Check sheet for the modelled part. Datum: model origin and axes. Units: mm. Face numbers are marked on the shaded views. A direction names the side the tool comes from. Round coordinates to 2 decimals unless told otherwise and drop trailing zeros. Write each loop counter-clockwise with the first axis right and the second up, starting at its lowest first coordinate (ties: lowest second). Pieces come first, ordered by that corner, then holes. Notation, with made-up numbers: M -12.75,64 L 7.25,64 A15 ccw 7.25,84 Z; hole C 52.25,-15 d1. An arc over 180 degrees is marked long. One line per item, written item: value.
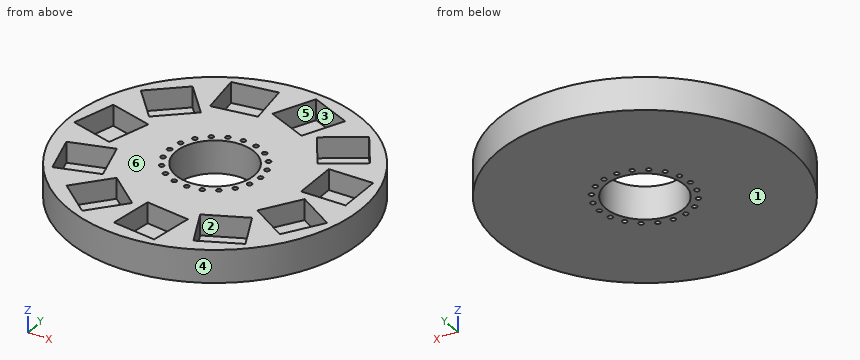
Autodesk Inventor part; units mm, degrees
ref_plane "YZ Plane" through (0, 0, 0) normal (1, 0, 0) x (0, 1, 0)
ref_plane "XZ Plane" through (0, 0, 0) normal (0, 1, 0) x (-1, 0, 0)
ref_plane "XY Plane" through (0, 0, 0) normal (0, 0, 1) x (1, 0, 0)
sketch "Sketch1" plane through (0, 0, 0) normal (0, 0, 1) x (1, 0, 0)
  circle A0 centre (0, 0) radius 45
  circle A1 centre (0, 0) radius 12
  dimension "d0" = 90
  dimension "d1" = 24
extrude "Extrusion1" add sketch "Sketch1" along normal blind 10
sketch "Sketch2" plane through (0, 0, 10) normal (0, 0, 1) x (1, 0, 0)
  line L0 (27.3, 12.7) -> (40, 12.7)
  line L1 (40, 12.7) -> (40, 0)
  line L2 (40, 0) -> (27.3, 0)
  line L3 (27.3, 0) -> (27.3, 12.7)
  line L4 (40.5, 13.2) -> (26.8, 13.2)
  line L5 (26.8, 13.2) -> (26.8, -0.5)
  line L6 (26.8, -0.5) -> (40.5, -0.5)
  line L7 (40.5, -0.5) -> (40.5, 13.2)
  point P0 (0, 0)
  dimension "d4" = 12.7
  dimension "d5" = 12.7
  dimension "d6" = 40
  dimension "d7" = 0.5
extrude "Extrusion2" cut sketch "Sketch2" against normal blind 6.35 contours L0 L1 L2 L3 | L7 L6 L5 L4
pattern_circular "Circular Pattern1" count 11 over 360 about axis through (0, 0, 0) along (0, 0, 1) of "Extrusion2"
sketch "Sketch3" plane through (0, 0, 10) normal (0, 0, 1) x (1, 0, 0)
  circle A0 centre (20, 0) radius 1.75
  circle A1 centre (14.1421, 14.1421) radius 1.75
  circle A2 centre (0, 20) radius 1.75
  circle A3 centre (-14.1421, 14.1421) radius 1.75
  circle A4 centre (-20, 0) radius 1.75
  circle A5 centre (-14.1421, -14.1421) radius 1.75
  circle A6 centre (0, -20) radius 1.75
  circle A7 centre (14.1421, -14.1421) radius 1.75
  point P0 (0, 0)
  dimension "d13" = 3.5
  dimension "d14" = 20
  dimension "d17" = 360
extrude "Extrusion3" [suppressed]
sketch "Sketch6" plane through (0, 0, 0) normal (0, 0, -1) x (-1, 0, 0)
  circle A0 centre (0, 14) radius 0.75
  circle A1 centre (-4.3262, 13.3148) radius 0.75
  circle A2 centre (-8.229, 11.3262) radius 0.75
  circle A3 centre (-11.3262, 8.229) radius 0.75
  circle A4 centre (-13.3148, 4.3262) radius 0.75
  circle A5 centre (-14, 0) radius 0.75
  circle A6 centre (-13.3148, -4.3262) radius 0.75
  circle A7 centre (-11.3262, -8.229) radius 0.75
  circle A8 centre (-8.229, -11.3262) radius 0.75
  circle A9 centre (-4.3262, -13.3148) radius 0.75
  circle A10 centre (0, -14) radius 0.75
  circle A11 centre (4.3262, -13.3148) radius 0.75
  circle A12 centre (8.229, -11.3262) radius 0.75
  circle A13 centre (11.3262, -8.229) radius 0.75
  circle A14 centre (13.3148, -4.3262) radius 0.75
  circle A15 centre (14, 0) radius 0.75
  circle A16 centre (13.3148, 4.3262) radius 0.75
  circle A17 centre (11.3262, 8.229) radius 0.75
  circle A18 centre (8.229, 11.3262) radius 0.75
  circle A19 centre (4.3262, 13.3148) radius 0.75
  point P0 (0, 0)
  dimension "d24" = 1.5
  dimension "d25" = 14
  dimension "d28" = 360
extrude "Extrusion5" cut sketch "Sketch6" against normal through all
properties part number "SG01" material "ABS Plastic"
Q1. Sectioned sample at B-B on z = 2. State how many separate pieces and enclosed holes the cut face has, and give its area (3 significant figures).
Completed:
separate pieces: 1
enclosed holes: 21
area: 5,870 mm^2
Q2. Access from +Z, -Z, +X, -X, +Y, -Y to the whole of each face (thin tool, end or side, straight path). Record for the marked faces 5 and 6.
Completed:
face 5: +Z
face 6: +Z, +X, -X, +Y, -Y
Q3. Scan lines: line 1 (Y direction, x = 31, z = 4.25); line 2 (X direction, y = -38, z = 5); line 3 (Y direction, x = -21.5, z = 7). Record each from-to range of solid material in increasing order. Write a range as [from, to].
Completed:
line 1: [-32.62, -20.52], [-4.23, -0.5], [13.2, 19.33], [26.67, 32.62]
line 2: [-24.1, -17.99], [-15.46, -5.97], [7.87, 24.1]
line 3: [-39.53, -34.96], [-24.05, 16.83], [25.58, 39.53]
Q4. Depth check by flat-ended pin: P1, Ø5.5, axis at x = 24, y = 22, coming from the +Z side; P2, Ø2, axis at x = 29, z = 7, coming from the -Y side; P3, Ø1.5, axis at x = 9, z = 9, coming from the +Y side. Enter the tip coordinate at first touch or a pass-through.
Completed:
P1: z = 3.65
P2: y = -35.23
P3: y = 44.24
Q5. Draft check along X on the marked faces 1, 2, 3 and 4. Enter one of: pulls with the +X half, pulls with the -X half, needs draft (parallel to the pull), parting line crosses it, or undercut.
Completed:
face 1: needs draft
face 2: undercut
face 3: undercut
face 4: parting line crosses it
Q6. Sectioned sample at A-A on y = 2.5. Enter the section's corners in (x, z).
Completed:
outline: M -44.93,0 L -11.74,0 L -11.74,10 L -27.2,10 L -27.2,3.65 L -41.48,3.65 L -41.48,10 L -44.93,10 Z; M 11.74,0 L 44.93,0 L 44.93,10 L 40.5,10 L 40.5,3.65 L 26.8,3.65 L 26.8,10 L 11.74,10 Z
